from build123d import *

# Parameters (mm, degrees)
EXTRUDE_1_DEPTH = 2.1


with BuildPart() as part:
    # Эскиз1 → Бобышка-Вытянуть1 (new body)
    with BuildSketch(Plane(origin=(0, 0, 0), x_dir=(-1, 0, 0), z_dir=(0, 0, -1))):
        with BuildLine():
            Line((-32.400001526, 25.399999619), (-29.75, 25.399999619))
            ThreePointArc((-29.75, 25.399999619), (-28.915971608, 25.747039587), (-28.575035851, 26.583581821))
            Line((-28.575035851, 26.583581821), (-28.575035851, 36.450190384))
            ThreePointArc((-28.575035851, 36.450190384), (-30.325030381, 38.200184914), (-28.575035851, 39.950179444))
            Line((-28.575035851, 39.950179444), (-28.575035851, 49.908417469))
            ThreePointArc((-28.575035851, 49.908417469), (-28.914981331, 50.715971039), (-29.725000381, 51.049999237))
            Line((-29.725000381, 51.049999237), (-32.400001526, 51.049999237))
            ThreePointArc((-32.400001526, 51.049999237), (-33.213001251, 50.713001251), (-33.549999237, 49.900001526))
            Line((-33.549999237, 49.900001526), (-33.549999237, 26.549999237))
            ThreePointArc((-33.549999237, 26.549999237), (-33.213000972, 25.736999232), (-32.400001526, 25.399999619))
        make_face()
    extrude(amount=-EXTRUDE_1_DEPTH)


solid = part.part
For this review, take the finished solid that the model builds, in its own axes (mm). Give positions to 0.01 mm unless a question says otherwise; leave off trailing zeros. Loops run counter-clockwise (first coordinate to the right, second up) from the corner with the lowest first, then second, coordinate; pieces in that order, holes last.
Item 1: Take a section at C-C, the plane y = 38.5. State the section outline as (x, z) points, and give its area (3 significant figures).
Item 2: Take a section at A-A, the plane x = 29.35. State the section outline as (y, z) points, and give its area (3 significant figures).
Item 3: For line 1 along Y through (x, z) = (30.1, 0.6); line 2 along Y through (x, z) = (28.8, 1.65); line 3 along Y through (x, z) = (32.8, 0.95), list the stretches that pass through material, from the lowest coordinate up.
Item 4: Draft analysis for pull direction Y (two halves, no side actions). For faces 1 (the cylindrical face through (33.204, 50.722, 1.035)), 2 (the cylindrical face through (30.325, 38.162, 1.035)), 3 (the flat face through (33.55, 38, 1)), state which applies: +Y half, -Y half, draft (parallel to the pull), parting line (faces both ways), or undercut.
Calculated:
1. outline: (30.3, 0) - (33.55, 0) - (33.55, 2.1) - (30.3, 2.1) - close
1. area: 6.83 mm2
2. outline: (25.47, 0) - (36.63, 0) - (36.63, 2.1) - (25.47, 2.1) - close; (39.77, 0) - (50.99, 0) - (50.99, 2.1) - (39.77, 2.1) - close
2. area: 47.0 mm2
3. line 1: y = 25.4 to 37.34, 39.06 to 51.05
3. line 2: y = 25.88 to 36.46, 39.94 to 50.58
3. line 3: y = 25.47 to 50.98
4. face 1: +Y half
4. face 2: undercut
4. face 3: draft
